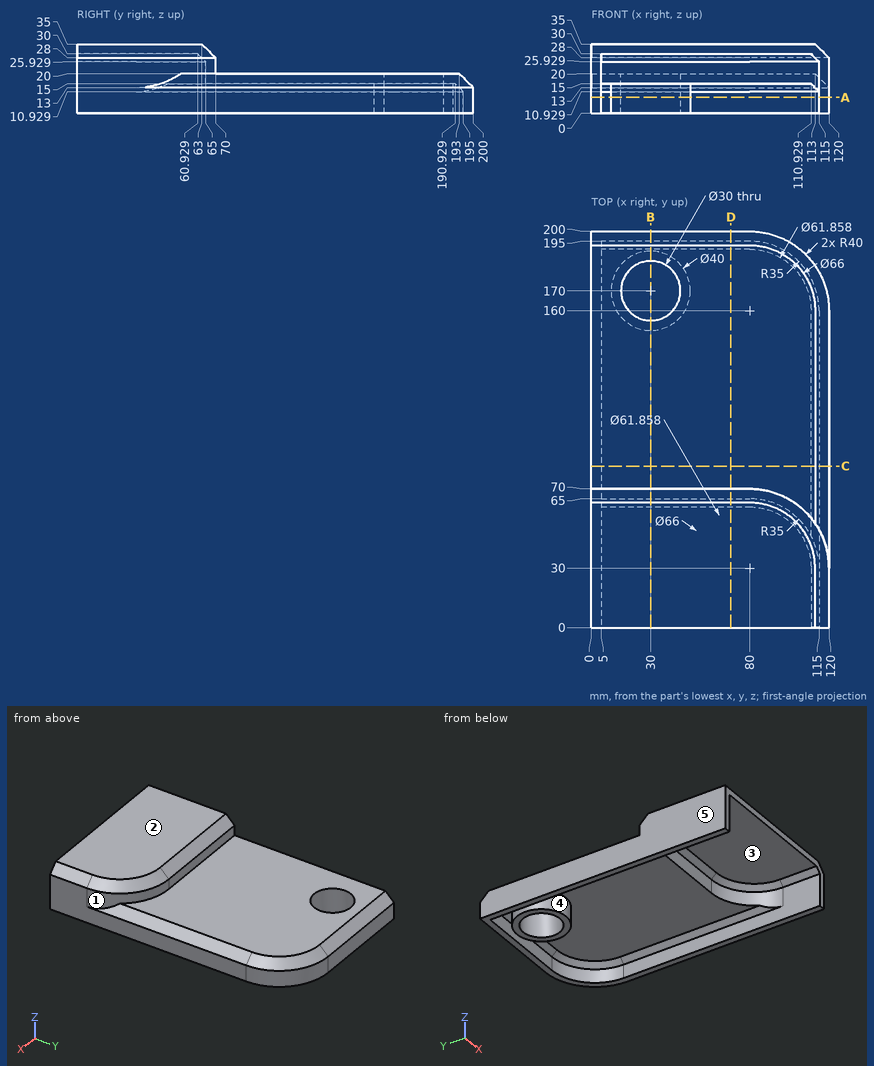
Verification items for this drawing (mm, ordinates from the low corner). A direction names the side the tool comes from. Coordinates: 2 decimals unless noted, no trailing zeros. Order: outer loops, then holes, each group sorted by start corner. A loop starts at its lowest first (then second) coordinate and runs counter-clockwise, first axis right, second up. Notation, with made-up numbers: M 2,12 L 50,12 A10 cw 50,19 Z; hole C -28.75,32 d11. An arc over 180 degrees is marked long. One line per item, written item: value. Start each with the question number.
Item 1: Depth check by flat-ended pin: P1, Ø12, axis at x = 47, z = 21, coming from the -Y side; P2, Ø9, axis at y = 120, z = 18, coming from the +X side; P3, Ø8.5, axis at x = 46.5, z = 3, coming from the -Y side. Enter the tip coordinate at first touch or a pass-through.
Item 2: Sectioned sample at A-A on z = 8. Record the cut outline in (x, y), then the cut area to 3 significant figures.
Item 3: Thickness scan on probe 1 along Y at (x, z) = (30, 8); probe 2 along Y at (x, z) = (35, 4.5) (1 decimal); probe 3 along X at (y, z) = (135, 9.5). Record the ranges inside material, lowest first.
Item 4: Sectioned sample at D-D on x = 70.5. Record the cut outline in (y, z), then the cut area to 3 significant figures.
Item 5: Access from +Z, -Z, +X, -X, +Y, -Y to the whole of each face (thin tool, end or side, straight path). Record for the marked faces 1, 2, 3, 4 and 5.
Item 6: Sectioned sample at C-C on y = 81.5. Record the cut outline in (x, z), then the cut area to 3 significant figures.
Item 7: Sectioned sample at B-B on x = 30. Record the cut outline in (y, z).
Calculated:
1. P1: y = 63.93
1. P2: x = 119.5
1. P3: y = 154.19
2. outline: M 0,0 L 5,0 L 5,195 L 80,195 A35 cw 115,160 L 115,0 L 120,0 L 120,160 A40 ccw 80,200 L 0,200 Z; C 30,170 d40; hole C 30,170 d30
2. area: 3,020 mm^2
3. probe 1: 150 to 155, 185 to 190, 195 to 200
3. probe 2: 150.6 to 155.9, 184.1 to 189.4, 195 to 200
3. probe 3: 0 to 5, 115 to 120
4. outline: M 0,30 L 60.93,30 L 65,25.93 L 65,15 L 190.93,15 L 195,10.93 L 195,0 L 200,0 L 200,13 L 193,20 L 70,20 L 70,28 L 63,35 L 0,35 Z
4. area: 1,120 mm^2
5. face 1: +Z, +X, +Y
5. face 2: +Z, +X, -X, +Y, -Y
5. face 3: -Z, -Y
5. face 4: -Z
5. face 5: +Z, -Z, -X, +Y, -Y
6. outline: M 0,0 L 5,0 L 5,15 L 110.93,15 L 115,10.93 L 115,0 L 120,0 L 120,13 L 113,20 L 0,20 Z
6. area: 734 mm^2
7. outline: M 0,30 L 60.93,30 L 65,25.93 L 65,15 L 150,15 L 150,0 L 155,0 L 155,20 L 70,20 L 70,28 L 63,35 L 0,35 Z; M 185,0 L 190,0 L 190,15 L 190.93,15 L 195,10.93 L 195,0 L 200,0 L 200,13 L 193,20 L 185,20 Z
